```python
from build123d import *

# Parameters (mm, degrees)
BOSS_EXTRUDE1_DEPTH = 1631.95
CUT_EXTRUDE2_DEPTH  = 76.2
SKETCH11_W          = 116.748947554
SKETCH11_H          = 157.612376209
CUT_EXTRUDE3_DEPTH  = 76.2


with BuildPart() as part:
    # Sketch1 → Boss-Extrude1 (new body)
    with BuildSketch(Plane.XY):
        with BuildLine():
            Line((-43.879451284, -42.2312162), (-48.35985275, -37.73138257))
            Line((-48.35985275, -37.73138257), (-3.361516443, 7.07263209))
            ThreePointArc((-3.361516443, 7.07263209), (1.150121774, 8.929986414), (5.653679589, 7.053124274))
            Line((5.653679589, 7.053124274), (50.457694249, -37.945212032))
            Line((50.457694249, -37.945212032), (45.957860619, -42.425613498))
            Line((45.957860619, -42.425613498), (2.869929296, 0.849196564))
            ThreePointArc((2.869929296, 0.849196564), (1.073761457, 1.597033186), (-0.724615856, 0.854525573))
            Line((-0.724615856, 0.854525573), (-43.879451284, -42.2312162))
        make_face()
    extrude(amount=BOSS_EXTRUDE1_DEPTH)

    # Sketch10 → Cut-Extrude2 (cut)
    with BuildSketch(Plane(origin=(-1.739591993, -803.922021371, 927.063003524), x_dir=(0.999998995, -0.000928778, 0.001071044), z_dir=(-0.001417661, -0.655147382, 0.755499767))):
        Polygon((-72.388022704, 958.296853766), (-72.388022704, 1089.35007065), (76.019748324, 1091.938631218), (76.019748324, 958.296853766), align=None)
    extrude(amount=CUT_EXTRUDE2_DEPTH, mode=Mode.SUBTRACT)

    # Sketch11 → Cut-Extrude3 (cut)
    with BuildSketch(Plane(origin=(0.008296278, 3.83397994, 4.421250898), x_dir=(0.999998995, -0.000928778, -0.001071044), z_dir=(0.001417661, 0.655147382, 0.755499767))):
        with Locations((-6.183779703, -23.975283789)):
            Rectangle(SKETCH11_W, SKETCH11_H)
    extrude(amount=-CUT_EXTRUDE3_DEPTH, mode=Mode.SUBTRACT)


solid = part.part
```
Here's how the part is built. I have some questions about the finished solid (model axes, mm). Give positions to 0.01 mm unless a question says otherwise; leave off trailing zeros. Loops run counter-clockwise (first coordinate to the right, second up) from the corner with the lowest first, then second, coordinate; pieces in that order, holes last. Notation, with made-up numbers: (-4, 63) -> (5, 63) arc R30 cw to (5, 96) -> close; hole circle Ø4 at (81.5, -31.75). An arc over 180 degrees is marked (long way). Use one line per item in the form item = value. Start each with the question number.
1) Thinking about a two-plate mould opening in X: for faces 1 (the face through (27.74, -15.13, 804.57)), 2 (the face through (-22, -20.387, 804.649)), 3 (the face through (-26.176, -15.643, 804.574)), which applies, +X half, -X half, draft (parallel to the pull), parting line (faces both ways), or undercut?
2) Imagine slicing it at B-B (z = 1375). Please give me the cut outline in (x, y).
3) Please list where these lines run through material, in increasing order: line 1 along Z through (x, y) = (-5, 1); line 2 along Y through (x, z) = (2.5, 1482.5); line 3 along X through (y, z) = (-1, 1132.5).
4) Imagine slicing it at A-A (y = -9). Please give me the cut outline in (x, z), then the cut area to 3 significant figures.
5) For P1, Ø1, axis at y = -23, z = 464.5, coming from the +X side; P2, Ø5, axis at y = -31.5, z = 1027.5, coming from the +X side; P3, Ø2, axis at y = -30, z = 680, coming from the +X side, each with a flat end and sliding along its axis, tell me the tip position at first contact or that it passes through.
Check values:
q1.face_1 = +X half
q1.face_2 = undercut
q1.face_3 = -X half
q2.outline = (-48.36, -37.73) -> (-43.88, -42.23) -> (-0.72, 0.85) arc R2.54 cw to (2.87, 0.85) -> (45.96, -42.43) -> (50.46, -37.95) -> (5.65, 7.05) arc R6.37 ccw to (-3.36, 7.07) -> close
q3.line_1 = 6.89 to 1625.06
q3.line_2 = 1.16 to 8.78
q3.line_3 = -11.47 to -2.58, 4.71 to 13.67
q4.outline = (-19.5, 15.59) -> (-10.59, 15.57) -> (-10.59, 1616.38) -> (-19.5, 1616.36) -> close; (12.68, 15.53) -> (21.64, 15.51) -> (21.64, 1616.44) -> (12.68, 1616.42) -> close
q4.area = 28,600 mm^2
q5.P1 = 36.07
q5.P2 = 46.53
q5.P3 = 43.54
